Check sheet for the modelled part. Datum: model origin and axes. Units: mm. A direction names the side the tool comes from. Round coordinates to 2 decimals unless told otherwise and drop trailing zeros. Write each loop counter-clockwise with the first axis right and the second up, starting at its lowest first coordinate (ties: lowest second). Pieces come first, ordered by that corner, then holes. Notation, with made-up numbers: (77.25, 63) - (84.25, 63) arc R17 ccw to (84.25, 93) - close; hole circle Ø4 at (42.25, 5). An arc over 180 degrees is marked (long way). Answer as a JSON object with one key per item and string values. Group by question number.
Item 1: Gauge pin test, flat ends, axial feed: P1, Ø1, axis at y = -6.5, z = -24, coming from the -X side; P2, Ø4, axis at y = -19.5, z = -10, coming from the +X side; P3, Ø3, axis at x = 208, z = 62.5, coming from the -Y side. Record the tip position at first contact, or that the pin passes through.
Item 2: Sectioned sample at A-A on x = 145. Record the boundary of the cut face in (y, z), plus the area to 3 significant figures.
Item 3: Sectioned sample at B-B on z = 18. Record the boundary of the cut face in (x, y).
Item 4: Set-up check for faces 1 (the cylindrical face through (130.26, -34.79, -188.48)), 2 (the flat face through (145, -50, -202)): record each of +Z, -Z, +X, -X, +Y, -Y from which the full face is reachable in a straight line by a thin tool's end or side.
Item 5: Thickness scan on line 1 (Y direction, x = 102, z = -19); line 2 (Z direction, x = 161, y = -4.5); line 3 (Z direction, x = 142.5, y = -24.5). Record the ranges inside material, lowest first.
Item 6: Sectioned sample at C-C on y = -45.5. Record the boundary of the cut face in (x, z).
Item 7: Release check for a two-part mould opening along X. For faces 3 (the flat face through (9, -10, 99)), 4 (the cylindrical face through (228.97, -34.79, 93.23)), 5 (the flat face through (143, 0, -29)) record: pulls with the +X half, pulls with the -X half, needs draft (parallel to the pull), parting line crosses it, or undercut.
```python
from build123d import *

# Parameters (mm, degrees)
F1_DEPTH = 20
F2_R     = 20
F3_DEPTH = 30


with BuildPart() as f1:
    # F0 (on Front) → F1 (new body)
    with BuildSketch(Plane.XZ):
        with BuildLine():
            add(Edge.make_bspline(
                [(0, 0), (15.8393937026, -64.3749522899), (73.9196968513, -158.1874761449), (132, -252)],
                knots=[0.3599862205, 0.3599862205, 0.3599862205, 0.3599862205, 1, 1, 1, 1], degree=3))
            Line((132, -252), (158, -252))
            add(Edge.make_bspline(
                [(290, 0), (274.1606062974, -64.3749522899), (216.0803031487, -158.1874761449), (158, -252)],
                knots=[0.3599862205, 0.3599862205, 0.3599862205, 0.3599862205, 1, 1, 1, 1], degree=3))
            Line((290, 0), (290, 90))
            Line((290, 90), (272, 108))
            Line((272, 108), (18, 108))
            Line((18, 108), (0, 90))
            Line((0, 90), (0, 0))
        make_face()
    extrude(amount=F1_DEPTH)

    # F2 (on face) → F3 (join)
    with BuildSketch(Plane.XZ.offset(20)):
        with Locations((46.2842712475, 79.7157287525)):
            Circle(F2_R)
        with Locations((243.7157287525, 79.7157287525)):
            Circle(F2_R)
        with Locations((145, -202)):
            Circle(F2_R)
    extrude(amount=F3_DEPTH)


solid = f1.part
```
Completed:
{
 "1": {"P1": "x = 7.14", "P2": "x = 287.86", "P3": "y = -20"},
 "2": {"outline": "(-50, -222) - (-20, -222) - (-20, -252) - (0, -252) - (0, 108) - (-20, 108) - (-20, -182) - (-50, -182) - close", "area": "8,400 mm²"},
 "3": {"outline": "(0, -20) - (290, -20) - (290, 0) - (0, 0) - close"},
 "4": {"face 1": "-Y", "face 2": "+Z, -Z, +X, -X, -Y"},
 "5": {"line 1": "-20 to 0", "line 2": "-247.15 to 108", "line 3": "-221.84 to -182.16"},
 "6": {"outline": "circle Ø40 at (46.28, 79.72); circle Ø40 at (145, -202); circle Ø40 at (243.72, 79.72)"},
 "7": {"face 3": "pulls with the -X half", "face 4": "undercut", "face 5": "needs draft"}
}
